Can you work these out from the model? Positions are in its coordinate system, mm. Face numbers are marked on the shaded views. A direction names the side the tool comes from. Coordinates: 2 decimals unless noted, no trailing zeros. Order: outer loops, then holes, each group sorted by start corner. A loop starts at its lowest first (then second) coordinate and runs counter-clockwise, first axis right, second up. Notation, with made-up numbers: M 57.25,51.5 L 63.25,51.5 A10 ccw 63.25,70.5 Z; hole C 29.5,33.25 d2. An arc over 180 degrees is marked long. Answer as CSV lines item,"result". Start each with the question number.
1. If we mould it in two halves opening along X, with no side actions, what happens to the marked faces 3 and 4? For each: released by +X, released by -X, zero draft, split by the parting line, or undercut.
2. If we section it at C-C (y = 1.27): Give the number of separate pieces and of enclosed holes in the cut face, plus the area to 3 significant figures.
3. I need wall thicknesses on line 1 along Y through (x, z) = (41.91, 0.05); line 2 along X through (y, z) = (14.25, -1.1); line 3 along Y through (x, z) = (50, -0.2). Which ranges of each line are inside material? Lowest first, please. Write a range as from..to.
4. On a 3-axis mill with a long thin cutter (end or side, diameter ignored), from which of +Z, -Z, +X, -X, +Y, -Y can I reach the whole of each face in a straight line? I mean the marked faces 1 and 2. Say none if no direction works.
5. If we section it at B-B (x = 41.91): List the corners of the cut face in (y, z) for me.
6. Will these pins go through, and if not, where does the flat tip stop? pin 1 (1.6 mm diameter, centred on x = 31.75, y = 1.27, fed in from -Z); pin 2 (6 mm diameter, centred on x = 27.5, y = 11.5, fed in from -Z); pin 3 (0.8 mm diameter, centred on x = 36.83, y = 21.59, fed in from +Z); pin 4 (0.7 mm diameter, centred on y = 14.5, z = -1.5, fed in from +X).
7. If we section it at A-A (z = -1.1): List the corners of the cut face in (x, y) for me, plus the area to 3 significant figures.
8. If we section it at D-D (x = 26.67): List the corners of the cut face in (y, z) for me.
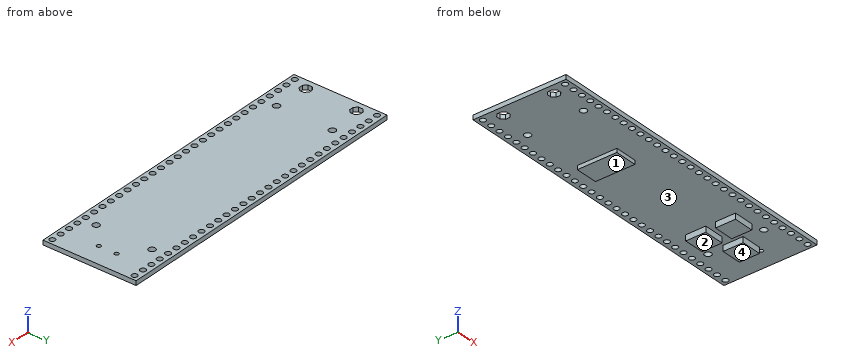
```python
from build123d import *

# Parameters (mm, degrees)
MAIN_BOARD_DEPTH      = 0.5461
MAIN_BOARD_DEPTH_BACK = 0.5461
SKETCH1_W             = 76.2
SKETCH1_H             = 23.0000048
SKETCH1_R             = 0.6858
SKETCH1_R_2           = 0.824992
SKETCH1_R_3           = 0.508
SKETCH2_W             = 4.953
SKETCH2_H             = 4.953
BUTTONS_ON_BACK_DEPTH = 1.397
SKETCH3_W             = 5.4864
SKETCH3_H             = 9.7536
CHIP_ON_BACK_DEPTH    = 0.9398


with BuildPart() as part:
    # Sketch1 → Main board (new, two sides: drawn at the far end of the back side and taken through both)
    with BuildSketch(Plane.XY.offset(-MAIN_BOARD_DEPTH_BACK)):
        with Locations((38.1, 11.5000024)):
            Rectangle(SKETCH1_W, SKETCH1_H)
        with Locations((1.27, 21.59)):
            Circle(SKETCH1_R, mode=Mode.SUBTRACT)
        with Locations((3.81, 21.59)):
            Circle(SKETCH1_R, mode=Mode.SUBTRACT)
        with Locations((6.35, 21.59)):
            Circle(SKETCH1_R, mode=Mode.SUBTRACT)
        with Locations((8.89, 21.59)):
            Circle(SKETCH1_R, mode=Mode.SUBTRACT)
        with Locations((11.43, 21.59)):
            Circle(SKETCH1_R, mode=Mode.SUBTRACT)
        with Locations((13.97, 21.59)):
            Circle(SKETCH1_R, mode=Mode.SUBTRACT)
        with Locations((16.51, 21.59)):
            Circle(SKETCH1_R, mode=Mode.SUBTRACT)
        with Locations((19.05, 21.59)):
            Circle(SKETCH1_R, mode=Mode.SUBTRACT)
        with Locations((21.59, 21.59)):
            Circle(SKETCH1_R, mode=Mode.SUBTRACT)
        with Locations((24.13, 21.59)):
            Circle(SKETCH1_R, mode=Mode.SUBTRACT)
        with Locations((26.67, 21.59)):
            Circle(SKETCH1_R, mode=Mode.SUBTRACT)
        with Locations((29.21, 21.59)):
            Circle(SKETCH1_R, mode=Mode.SUBTRACT)
        with Locations((31.75, 21.59)):
            Circle(SKETCH1_R, mode=Mode.SUBTRACT)
        with Locations((34.29, 21.59)):
            Circle(SKETCH1_R, mode=Mode.SUBTRACT)
        with Locations((36.83, 21.59)):
            Circle(SKETCH1_R, mode=Mode.SUBTRACT)
        with Locations((39.37, 21.59)):
            Circle(SKETCH1_R, mode=Mode.SUBTRACT)
        with Locations((41.91, 21.59)):
            Circle(SKETCH1_R, mode=Mode.SUBTRACT)
        with Locations((44.45, 21.59)):
            Circle(SKETCH1_R, mode=Mode.SUBTRACT)
        with Locations((46.99, 21.59)):
            Circle(SKETCH1_R, mode=Mode.SUBTRACT)
        with Locations((49.53, 21.59)):
            Circle(SKETCH1_R, mode=Mode.SUBTRACT)
        with Locations((52.07, 21.59)):
            Circle(SKETCH1_R, mode=Mode.SUBTRACT)
        with Locations((54.61, 21.59)):
            Circle(SKETCH1_R, mode=Mode.SUBTRACT)
        with Locations((57.15, 21.59)):
            Circle(SKETCH1_R, mode=Mode.SUBTRACT)
        with Locations((59.69, 21.59)):
            Circle(SKETCH1_R, mode=Mode.SUBTRACT)
        with Locations((62.23, 21.59)):
            Circle(SKETCH1_R, mode=Mode.SUBTRACT)
        with Locations((64.77, 21.59)):
            Circle(SKETCH1_R, mode=Mode.SUBTRACT)
        with Locations((67.31, 21.59)):
            Circle(SKETCH1_R, mode=Mode.SUBTRACT)
        with Locations((69.85, 21.59)):
            Circle(SKETCH1_R, mode=Mode.SUBTRACT)
        with Locations((72.39, 21.59)):
            Circle(SKETCH1_R, mode=Mode.SUBTRACT)
        with Locations((74.93, 21.59)):
            Circle(SKETCH1_R, mode=Mode.SUBTRACT)
        with Locations((65.5999958, 18.2999888)):
            Circle(SKETCH1_R_2, mode=Mode.SUBTRACT)
        with Locations((65.5999958, 4.499991)):
            Circle(SKETCH1_R_2, mode=Mode.SUBTRACT)
        with Locations((10.8000038, 18.2999888)):
            Circle(SKETCH1_R_2, mode=Mode.SUBTRACT)
        with Locations((10.8000038, 4.499991)):
            Circle(SKETCH1_R_2, mode=Mode.SUBTRACT)
        with Locations((71.0499976, 13.9999974)):
            Circle(SKETCH1_R_3, mode=Mode.SUBTRACT)
        with Locations((71.0499976, 9.6000062)):
            Circle(SKETCH1_R_3, mode=Mode.SUBTRACT)
        with Locations((1.27, 1.27)):
            Circle(SKETCH1_R, mode=Mode.SUBTRACT)
        with Locations((3.81, 1.27)):
            Circle(SKETCH1_R, mode=Mode.SUBTRACT)
        with Locations((6.35, 1.27)):
            Circle(SKETCH1_R, mode=Mode.SUBTRACT)
        with Locations((8.89, 1.27)):
            Circle(SKETCH1_R, mode=Mode.SUBTRACT)
        with Locations((11.43, 1.27)):
            Circle(SKETCH1_R, mode=Mode.SUBTRACT)
        with Locations((13.97, 1.27)):
            Circle(SKETCH1_R, mode=Mode.SUBTRACT)
        with Locations((16.51, 1.27)):
            Circle(SKETCH1_R, mode=Mode.SUBTRACT)
        with Locations((19.05, 1.27)):
            Circle(SKETCH1_R, mode=Mode.SUBTRACT)
        with Locations((21.59, 1.27)):
            Circle(SKETCH1_R, mode=Mode.SUBTRACT)
        with Locations((24.13, 1.27)):
            Circle(SKETCH1_R, mode=Mode.SUBTRACT)
        with Locations((26.67, 1.27)):
            Circle(SKETCH1_R, mode=Mode.SUBTRACT)
        with Locations((29.21, 1.27)):
            Circle(SKETCH1_R, mode=Mode.SUBTRACT)
        with Locations((31.75, 1.27)):
            Circle(SKETCH1_R, mode=Mode.SUBTRACT)
        with Locations((34.29, 1.27)):
            Circle(SKETCH1_R, mode=Mode.SUBTRACT)
        with Locations((36.83, 1.27)):
            Circle(SKETCH1_R, mode=Mode.SUBTRACT)
        with Locations((39.37, 1.27)):
            Circle(SKETCH1_R, mode=Mode.SUBTRACT)
        with Locations((41.91, 1.27)):
            Circle(SKETCH1_R, mode=Mode.SUBTRACT)
        with Locations((44.45, 1.27)):
            Circle(SKETCH1_R, mode=Mode.SUBTRACT)
        with Locations((46.99, 1.27)):
            Circle(SKETCH1_R, mode=Mode.SUBTRACT)
        with Locations((49.53, 1.27)):
            Circle(SKETCH1_R, mode=Mode.SUBTRACT)
        with Locations((52.07, 1.27)):
            Circle(SKETCH1_R, mode=Mode.SUBTRACT)
        with Locations((54.61, 1.27)):
            Circle(SKETCH1_R, mode=Mode.SUBTRACT)
        with Locations((59.69, 1.27)):
            Circle(SKETCH1_R, mode=Mode.SUBTRACT)
        with Locations((57.15, 1.27)):
            Circle(SKETCH1_R, mode=Mode.SUBTRACT)
        with Locations((62.23, 1.27)):
            Circle(SKETCH1_R, mode=Mode.SUBTRACT)
        with Locations((64.77, 1.27)):
            Circle(SKETCH1_R, mode=Mode.SUBTRACT)
        with Locations((69.85, 1.27)):
            Circle(SKETCH1_R, mode=Mode.SUBTRACT)
        with Locations((67.31, 1.27)):
            Circle(SKETCH1_R, mode=Mode.SUBTRACT)
        with Locations((72.39, 1.27)):
            Circle(SKETCH1_R, mode=Mode.SUBTRACT)
        with Locations((74.93, 1.27)):
            Circle(SKETCH1_R, mode=Mode.SUBTRACT)
        Polygon((3.769995, 16.97393862), (3.769995, 18.02604218), (3.02604678, 18.7699904), (1.97394322, 18.7699904), (1.229995, 18.02604218), (1.229995, 16.97393862), (1.97394322, 16.2299904), (3.02604678, 16.2299904), align=None, mode=Mode.SUBTRACT)
        Polygon((3.769995, 4.47393822), (3.769995, 5.52604178), (3.02604678, 6.26999), (1.97394322, 6.26999), (1.229995, 5.52604178), (1.229995, 4.47393822), (1.97394322, 3.72999), (3.02604678, 3.72999), align=None, mode=Mode.SUBTRACT)
    extrude(amount=MAIN_BOARD_DEPTH + MAIN_BOARD_DEPTH_BACK)

    # Sketch2 → Buttons on back (add)
    with BuildSketch(Plane(origin=(0, 0, -0.5461), x_dir=(-1, 0, 0), z_dir=(0, 0, -1))):
        with Locations((-67.4243, 11.5573048)):
            Rectangle(SKETCH2_W, SKETCH2_H)
        with Locations((-60.0075, 14.7577048)):
            Rectangle(SKETCH2_W, SKETCH2_H)
        with Locations((-60.0075, 7.4295)):
            Rectangle(SKETCH2_W, SKETCH2_H)
    extrude(amount=BUTTONS_ON_BACK_DEPTH)

    # Sketch3 → Chip on back (add)
    with BuildSketch(Plane(origin=(0, 0, -0.5461), x_dir=(-1, 0, 0), z_dir=(0, 0, -1))):
        with Locations((-27.9908, 12.8908048)):
            Rectangle(SKETCH3_W, SKETCH3_H)
    extrude(amount=CHIP_ON_BACK_DEPTH)


solid = part.part
```
Solved:
1,face 3,"undercut"
1,face 4,"zero draft"
2,separate pieces,"31"
2,enclosed holes,"0"
2,area,"38.3 mm²"
3,line 1,"0..0.58, 1.96..20.9, 22.28..23"
3,line 2,"25.25..30.73, 57.53..62.48"
3,line 3,"0..0.77, 1.77..21.09, 22.09..23"
4,face 1,"-Z, -X, +Y, -Y"
4,face 2,"-Z, +X, -X, +Y, -Y"
5,outline,"M 0,-0.55 L 0.58,-0.55 L 0.58,0.55 L 0,0.55 Z; M 1.96,-0.55 L 20.9,-0.55 L 20.9,0.55 L 1.96,0.55 Z; M 22.28,-0.55 L 23,-0.55 L 23,0.55 L 22.28,0.55 Z"
6,pin 1,"z = -0.55"
6,pin 2,"z = -1.49"
6,pin 3,"through"
6,pin 4,"x = 62.48"
7,outline,"M 25.25,8.01 L 30.73,8.01 L 30.73,17.77 L 25.25,17.77 Z; M 57.53,4.95 L 62.48,4.95 L 62.48,9.91 L 57.53,9.91 Z; M 57.53,12.28 L 62.48,12.28 L 62.48,17.23 L 57.53,17.23 Z; M 64.95,9.08 L 69.9,9.08 L 69.9,14.03 L 64.95,14.03 Z"
7,area,"127 mm²"
8,outline,"M 0,-0.55 L 0.58,-0.55 L 0.58,0.55 L 0,0.55 Z; M 1.96,-0.55 L 8.01,-0.55 L 8.01,-1.49 L 17.77,-1.49 L 17.77,-0.55 L 20.9,-0.55 L 20.9,0.55 L 1.96,0.55 Z; M 22.28,-0.55 L 23,-0.55 L 23,0.55 L 22.28,0.55 Z"
